For this review, use the dimensioned drawing (mm, ordinates from the lowest corner) and the shaded views. Round coordinates to 2 decimals unless told otherwise and drop trailing zeros. Loops run counter-clockwise (first coordinate to the right, second up) from the corner with the lowest first, then second, coordinate; pieces in that order, holes last. Notation, with made-up numbers: M 39.5,17 L 64.5,17 A32 ccw 64.5,43 Z; hole C 21.5,14.5 d2. An arc over 180 degrees is marked long. Write item = value, one per line. Start each with the question number.
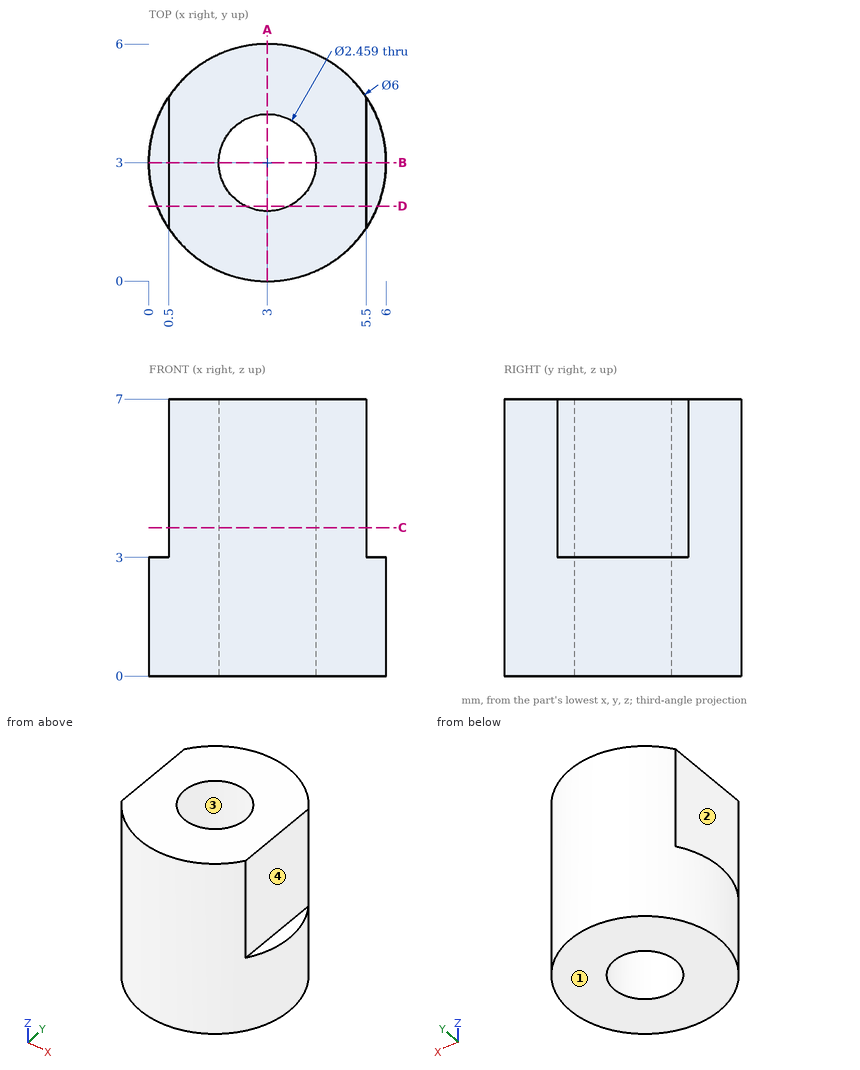
(1) Add section A-A on x = 3. Write out the cut boundary in (y, z).
(2) Add section B-B on y = 3. Write out the cut boundary in (x, z), and give its area (3 significant figures).
(3) For pin 1 Ø2.5 at (y, z) = (3, 4.5) entering from -X; pin 2 Ø1 at (x, z) = (2, 3) entering from +Y; pin 3 Ø1 at (y, z) = (3.5, 4) entering from +X, all flat-tipped, find the tip position at first contact; note any pin that passes through.
(4) Add section C-C on z = 3.75. Write out the cut boundary in (x, y).
(5) Add section D-D on y = 1.9. Write out the cut boundary in (x, z).
(6) Draft analysis for pull direction X (two halves, no side actions). For the marked faces 1, 2, 3 and 4, state which applies: +X half, -X half, draft (parallel to the pull), parting line (faces both ways), or undercut.
(7) Wall thickness on L1, parallel to X at y = 3, z = 1.75; L2, parallel to X at y = 3, z = 3.5: over which ranges is each line inside the solid? List them lowest first.
Answer sheet:
q1.outline = M 0,0 L 1.77,0 L 1.77,7 L 0,7 Z; M 4.23,0 L 6,0 L 6,7 L 4.23,7 Z
q2.outline = M 0,0 L 1.77,0 L 1.77,7 L 0.5,7 L 0.5,3 L 0,3 Z; M 4.23,0 L 6,0 L 6,3 L 5.5,3 L 5.5,7 L 4.23,7 Z
q2.area = 20.8 mm²
q3.pin_1 = 0.5
q3.pin_2 = 5.96
q3.pin_3 = 5.5
q4.outline = M 0.5,1.34 A3 ccw 5.5,1.34 L 5.5,4.66 A3 ccw 0.5,4.66 Z; hole C 3,3 d2.46
q5.outline = M 0.21,0 L 2.45,0 L 2.45,7 L 0.5,7 L 0.5,3 L 0.21,3 Z; M 3.55,0 L 5.79,0 L 5.79,3 L 5.5,3 L 5.5,7 L 3.55,7 Z
q6.face_1 = draft
q6.face_2 = -X half
q6.face_3 = undercut
q6.face_4 = +X half
q7.L1 = 0 to 1.77, 4.23 to 6
q7.L2 = 0.5 to 1.77, 4.23 to 5.5
